Could you check a few things on this model? Use its own coordinates, in mm. Face numbers are marked on the shaded views. A direction names the side the tool comes from. Coordinates: 2 decimals unless noted, no trailing zeros. Order: outer loops, then holes, each group sorted by start corner. A loop starts at its lowest first (then second) coordinate and runs counter-clockwise, first axis right, second up.
```python
from build123d import *

# Parameters (mm, degrees)
SKETCH1_W           = 12.7
SKETCH1_H           = 38.1
BOSS_EXTRUDE1_DEPTH = 155.575
SKETCH3_W           = 12.7
SKETCH3_H           = 38.1
BOSS_EXTRUDE2_DEPTH = 130.175
SKETCH4_W           = 100.6348
SKETCH4_H           = 12.192
BOSS_EXTRUDE3_DEPTH = 101.0412
CUT_EXTRUDE2_DEPTH  = 12.192
BOSS_EXTRUDE8_START = 61.0616
SKETCH6_R           = 44.45
SKETCH6_R_2         = 39.3192
BOSS_EXTRUDE8_DEPTH = 61.0616


with BuildPart() as part:
    # Sketch1 → Boss-Extrude1 (new body)
    with BuildSketch(Plane(origin=(0, 0, 0), x_dir=(0, -1, 0), z_dir=(-1, 0, 0))):
        with Locations((-6.35, 19.05)):
            Rectangle(SKETCH1_W, SKETCH1_H)
    extrude(amount=-BOSS_EXTRUDE1_DEPTH)

    # Sketch3 → Boss-Extrude2 (add)
    with BuildSketch(Plane(origin=(0, 12.7, 0), x_dir=(1, 0, 0), z_dir=(0, 1, 0))):
        with Locations((6.35, -19.05)):
            Rectangle(SKETCH3_W, SKETCH3_H)
    extrude(amount=BOSS_EXTRUDE2_DEPTH)

    # Sketch4 → Boss-Extrude3 (add)
    with BuildSketch(Plane(origin=(0, 12.7, 0), x_dir=(1, 0, 0), z_dir=(0, 1, 0))):
        with Locations((63.0174, -18.796)):
            Rectangle(SKETCH4_W, SKETCH4_H)
    extrude(amount=BOSS_EXTRUDE3_DEPTH)

    # Sketch5 → Cut-Extrude2 (cut)
    with BuildSketch(Plane.XY.offset(24.892)):
        Polygon((12.7, 58.42), (58.42, 12.7), (12.7, 12.7), align=None)
    extrude(amount=-CUT_EXTRUDE2_DEPTH, mode=Mode.SUBTRACT)

    # Sketch6 → Boss-Extrude8 (add)
    with BuildSketch(Plane(origin=(0, 0, 12.7), x_dir=(-1, 0, 0), z_dir=(0, 0, -1)).offset(BOSS_EXTRUDE8_START)):
        with Locations(Location((-57.2008, 57.2008, 0), (0, 0, 1.486934097))):
            Circle(SKETCH6_R)
        with Locations(Location((-57.2008, 57.2008, 0), (0, 0, 180))):
            Circle(SKETCH6_R_2, mode=Mode.SUBTRACT)
    extrude(amount=-BOSS_EXTRUDE8_DEPTH)


solid = part.part
```
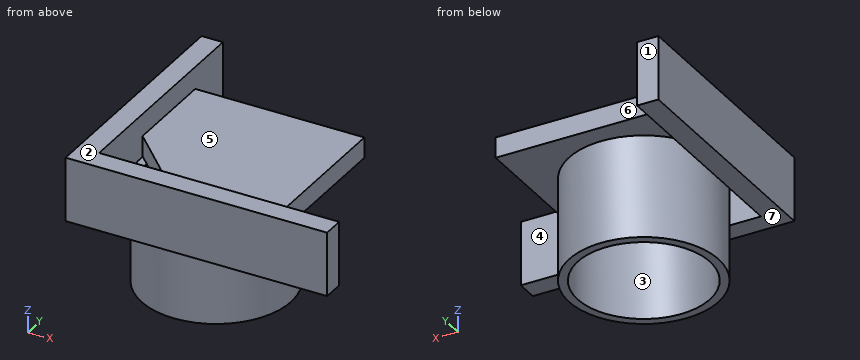
Item 1: Suppose I cut it at C-C (y = 39.5). List the corners of the cut face in (x, z) for me.
Item 2: I need wall thicknesses on line 1 (Z direction, x = 26, y = 28); line 2 (X direction, y = 22, z = 33); line 3 (X direction, y = 22.5, z = 3). Which ranges of each line are inside material? Lowest first, please.
Item 3: Suppose I cut it at B-B (x = 56). List the corners of the cut face in (y, z) for me, and give its area (3 significant figures).
Item 4: For pin 1 Ø12 at (x, y) = (54.5, 52.5) entering from +Z; pin 2 Ø4 at (y, z) = (24.5, 29) entering from +X; pin 3 Ø6 at (y, z) = (43, 19.5) entering from +X, each with a flat end and sliding along its axis, tell me the tip position at first contact or that it passes through.
Item 5: Thinking about a two-plate mould opening in Y: for the marked faces 1, 2 and 3, which applies, +Y half, -Y half, draft (parallel to the pull), parting line (faces both ways), or undercut?
Item 6: Which directions (+Z, -Z, +X, -X, +Y, -Y) give clear straight access to the entire face, cutting with the end or side of a thin tool? Please do the marked faces 4, 5, 6 and 7.
Item 7: Suppose I cut it at D-D (x = 111). List the corners of the cut face in (y, z) for me.
Item 8: Suppose I cut it at A-A (z = 8). List the corners of the cut face in (x, y) for me (3 decimals), and give its area (3 significant figures).
Geometry results:
1. outline: (0, 0) - (12.7, 0) - (12.7, 38.1) - (0, 38.1) - close; (16.43, -48.36) - (22.09, -48.36) - (22.09, 12.7) - (16.43, 12.7) - close; (31.62, 12.7) - (92.31, 12.7) - (92.31, -48.36) - (97.97, -48.36) - (97.97, 12.7) - (113.33, 12.7) - (113.33, 24.89) - (31.62, 24.89) - close
2. line 1: z = -48.36 to 12.7
2. line 2: x = 0 to 12.7
2. line 3: x = 0 to 12.7, 29.42 to 38.71, 75.69 to 84.98
3. outline: (0, 0) - (12.7, 0) - (12.7, 38.1) - (0, 38.1) - close; (12.77, -48.36) - (17.9, -48.36) - (17.9, 12.7) - (96.5, 12.7) - (96.5, -48.36) - (101.63, -48.36) - (101.63, 12.7) - (113.74, 12.7) - (113.74, 24.89) - (15.12, 24.89) - (15.12, 12.7) - (12.77, 12.7) - close
3. area: 2,310 mm2
4. pin 1: stops at z = 24.89
4. pin 2: stops at x = 12.7
4. pin 3: stops at x = 113.33
5. face 1: +Y half
5. face 2: draft
5. face 3: undercut
6. face 4: none
6. face 5: +Z, +X, +Y
6. face 6: +Z, -Z, +X, +Y
6. face 7: -Z, -X, -Y
7. outline: (0, 0) - (12.7, 0) - (12.7, 12.7) - (113.74, 12.7) - (113.74, 24.89) - (12.7, 24.89) - (12.7, 38.1) - (0, 38.1) - close
8. outline: (0, 0) - (155.575, 0) - (155.575, 12.7) - (12.7, 12.7) - (12.7, 142.875) - (0, 142.875) - close; circle Ø88.9 at (57.201, 57.201); hole circle Ø78.638 at (57.201, 57.201)
8. area: 4,980 mm2
